from build123d import *

# Parameters (mm, degrees)
F0_W     = 200
F0_H     = 400
F1_DEPTH = 200
F2_R     = 25
F3_DEPTH = 200.001
F4_R     = 63.5
F5_SIZE  = 63.5


with BuildPart() as f1:
    # F0 (on Front) → F1 (new body)
    with BuildSketch(Plane.XZ):
        Rectangle(F0_W, F0_H)
    extrude(amount=F1_DEPTH)

    # F2 (on face) → F3 (cut, through all)
    with BuildSketch(Plane.XZ.offset(200)):
        Circle(F2_R)
    extrude(amount=-F3_DEPTH, mode=Mode.SUBTRACT)

    # F4
    f4_edges = [f1.edges().sort_by_distance(p)[0] for p in [
        (100, -100, 200),
        (-100, -100, 200),
    ]]
    fillet(f4_edges, radius=F4_R)

    # F5
    f5_edges = [f1.edges().sort_by_distance(p)[0] for p in [
        (-100, -100, -200),
        (100, -100, -200),
    ]]
    chamfer(f5_edges, length=F5_SIZE)


solid = f1.part
Verification items for the finished model (mm, model axes). Round coordinates to 2 decimals unless told otherwise and drop trailing zeros. Loops run counter-clockwise (first coordinate to the right, second up) from the corner with the lowest first, then second, coordinate; pieces in that order, holes last. Notation, with made-up numbers: (-24, -38) - (2, -38) arc R33 ccw to (2, -2) - close; hole circle Ø6 at (46.5, 43). An arc over 180 degrees is marked (long way). Use one line per item in the form item = value.
1. Draft check along X on faces 1 (the cylindrical face through (-81.892, -101.4, 180.905)), 2 (the flat face through (-1, -200, 47)), 3 (the cylindrical face through (80.905, -101.4, 181.892)), 4 (the cylindrical face through (23.846, -101.4, 7.509)). Enter one of: pulls with the +X half, pulls with the -X half, needs draft (parallel to the pull), parting line crosses it, or undercut.
A:
face_1 = pulls with the -X half
face_2 = needs draft
face_3 = pulls with the +X half
face_4 = undercut
2. Section check B-B on y = -67.5. Record the cut outline in (x, z).
A:
outline = (-100, -136.5) - (-36.5, -200) - (36.5, -200) - (100, -136.5) - (100, 136.5) arc R63.5 ccw to (36.5, 200) - (-36.5, 200) arc R63.5 ccw to (-100, 136.5) - close; hole circle Ø50 at (0, 0)
3. Section check C-C on z = 0. Record the cut outline in (x, y).
A:
outline = (-100, -200) - (-25, -200) - (-25, 0) - (-100, 0) - close; (25, -200) - (100, -200) - (100, 0) - (25, 0) - close
4. Scan lines: probe 1 along Z at (x, y) = (0, -111.5); probe 2 along Z at (x, y) = (-8, -104); probe 3 along X at (y, z) = (-188, -21). Record each from-to range of solid material in increasing order.
A:
probe_1 = -200 to -25, 25 to 200
probe_2 = -200 to -23.69, 23.69 to 200
probe_3 = -100 to -13.56, 13.56 to 100
5. Section check A-A on x = 0. Record the cut outline in (y, z).
A:
outline = (-200, -200) - (0, -200) - (0, -25) - (-200, -25) - close; (-200, 25) - (0, 25) - (0, 200) - (-200, 200) - close
6. Section check D-D on z = -154. Record the cut outline in (x, y).
A:
outline = (-82.5, -200) - (82.5, -200) - (82.5, 0) - (-82.5, 0) - close
